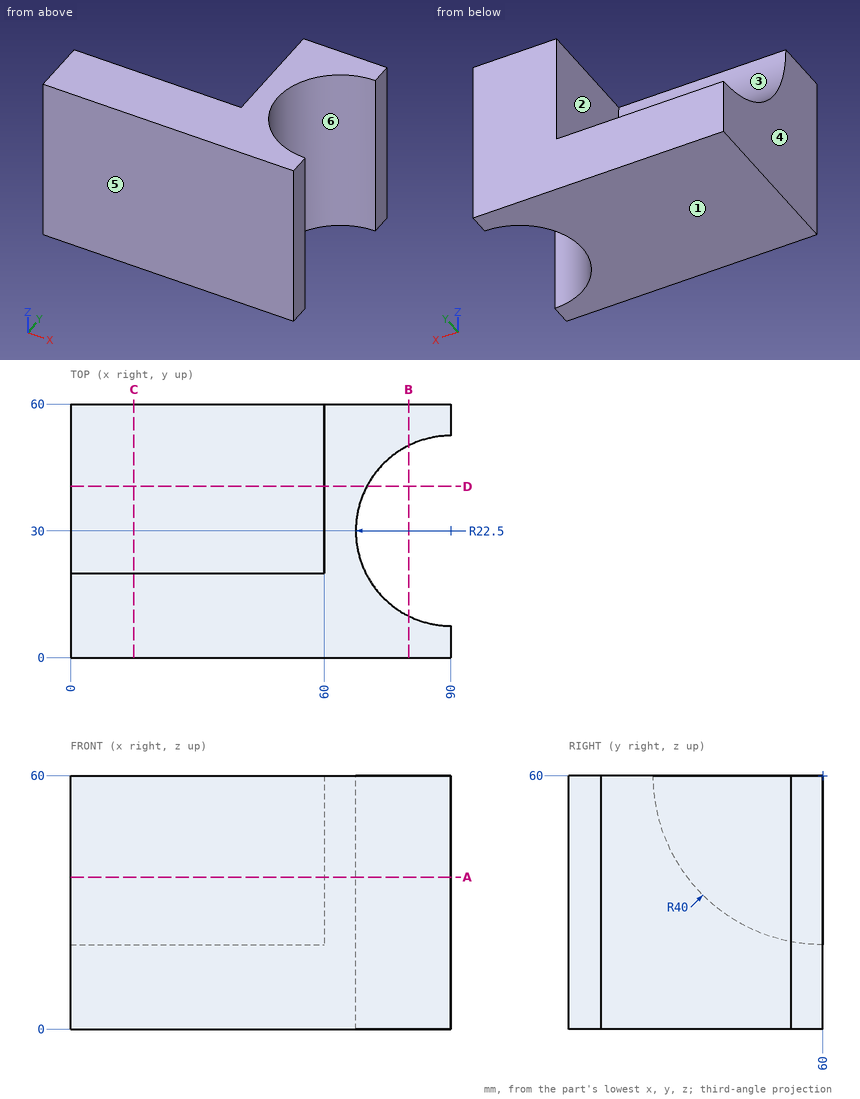
Drawing for the job (mm, zero at the part's lowest x, y, z). A direction names the side the tool comes from. Give positions to 0.01 mm unless a question says otherwise; leave off trailing zeros. Order: outer loops, then holes, each group sorted by start corner. A loop starts at its lowest first (then second) coordinate and runs counter-clockwise, first axis right, second up. Notation, with made-up numbers: (89, -13.5) -> (108, -13.5) arc R33 ccw to (108, 23.5) -> close; hole circle Ø1 at (53.5, 47.5). An arc over 180 degrees is marked (long way). Use one line per item in the form item = value.
(1) Tool access for the marked faces 1 and 2: list every direction of +Z, -Z, +X, -X, +Y, -Y with a clear straight run to the whole face (end or side of a thin tool).
Solution:
face_1 = -Z, +X, -X, +Y, -Y
face_2 = +Z, -X, +Y
(2) Saw through at A-A (z = 36). Write the cut outline in (x, y).
Solution:
outline = (0, 0) -> (90, 0) -> (90, 7.5) arc R22.5 cw to (90, 52.5) -> (90, 60) -> (60, 60) -> (60, 28) -> (0, 28) -> close
(3) Pull direction Y, two halves, no side cores. Call the marked faces 3, 4, 5 and 6: +Y half, -Y half, draft (parallel to the pull), parting line (faces both ways), or undercut.
Solution:
face_3 = +Y half
face_4 = draft
face_5 = -Y half
face_6 = undercut
(4) Saw through at B-B (x = 80). Write the cut outline in (y, z), then the cut area to 3 significant figures.
Solution:
outline = (0, 0) -> (9.84, 0) -> (9.84, 60) -> (0, 60) -> close; (50.16, 0) -> (60, 0) -> (60, 60) -> (50.16, 60) -> close
area = 1,180 mm²
(5) Saw through at D-D (y = 40.5). Write the cut outline in (x, z), then the cut area to 3 significant figures.
Solution:
outline = (0, 0) -> (70.1, 0) -> (70.1, 60) -> (60, 60) -> (60, 25.08) -> (0, 25.08) -> close
area = 2,110 mm²
(6) Flat gauge pins, fed straight in: P1, Ø1, axis at x = 44, z = 7.5, coming from the -Y side; P2, Ø12, axis at y = 18.5, z = 41.5, coming from the +X side; P3, Ø3, axis at y = 13, z = 8.5, coming from the +X side; P4, Ø4, axis at y = 33.5, z = 9.5, coming from the +X side. Where does each tip first touch, or does it go through?
Solution:
P1 = 0
P2 = 75.86
P3 = 77.19
P4 = 68.18
(7) Saw through at C-C (x = 15). Write the cut outline in (y, z).
Solution:
outline = (0, 0) -> (60, 0) -> (60, 20) arc R40 cw to (20, 60) -> (0, 60) -> close
(8) Drill centre lines: line 1 (Y direction, x = 71, z = 27); line 2 (X direction, y = 44.5, z = 25.5); line 3 (X direction, y = 18.5, z = 19.5). Where is each one in solid material? Low to high. Write a range as from..to.
Solution:
line_1 = 0..17.95, 42.05..60
line_2 = 60..72.8
line_3 = 0..70.66
